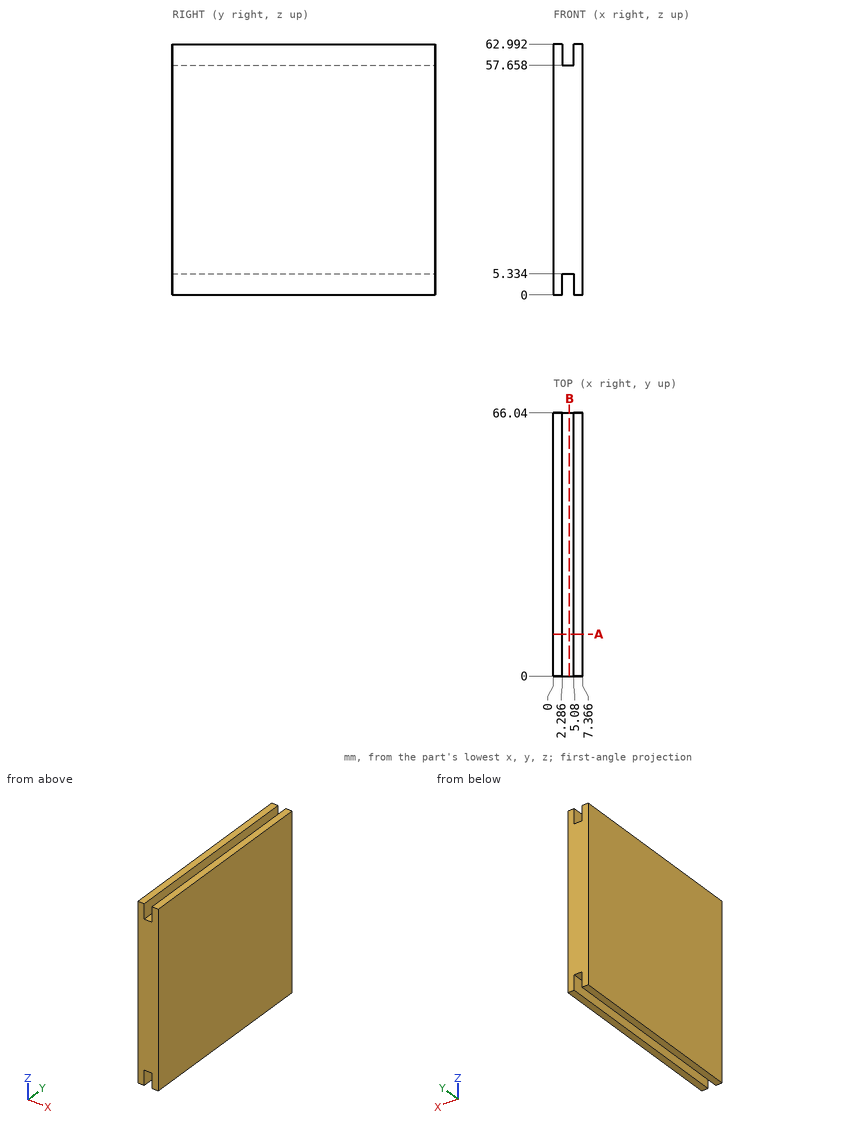
Here's the drawing with two shaded views (mm, measured from the low corner). I have some questions. Coordinates: 2 decimals unless noted, no trailing zeros. Write each loop counter-clockwise with the first axis right and the second up, starting at its lowest first coordinate (ties: lowest second). Pieces come first, ordered by that corner, then holes. Notation, with made-up numbers: (14, 87.25) -> (73, 87.25) arc R13 cw to (73, 107.25) -> close; hole circle Ø10 at (42.5, -25.75). An arc over 180 degrees is marked (long way). Use a Markdown table: item, result. Add a question column.
(1) If we section it at B-B, the plane x = 4: Write out the boundary of the cut face in (y, z).
(2) If we section it at A-A, the plane y = 10.5: Write out the boundary of the cut face in (x, z).
(3) I'm going to push a flat-ended pin straight in: P1, Ø0.8, axis at x = 4, y = 34, coming from the +Z side. Where does the tip first touch, or does it pass through?
(4) Please list where these lines run through material, in increasing order: line 1 (X direction, y = 39.5, z = 58); line 2 (Z direction, x = 3.5, y = 10.5).
Outcome:
| question | item | result |
|---|---|---|
| 1 | outline | (0, 5.33) -> (66.04, 5.33) -> (66.04, 57.66) -> (0, 57.66) -> close |
| 2 | outline | (0, 0) -> (2.29, 0) -> (2.29, 5.33) -> (5.08, 5.33) -> (5.08, 0) -> (7.37, 0) -> (7.37, 62.99) -> (5.08, 62.99) -> (5.08, 57.66) -> (2.29, 57.66) -> (2.29, 62.99) -> (0, 62.99) -> close |
| 3 | P1 | stops at z = 57.66 |
| 4 | line 1 | x = 0 to 2.29, 5.08 to 7.37 |
| 4 | line 2 | z = 5.33 to 57.66 |
